```python
from build123d import *

# Parameters (mm, degrees)
F1_DEPTH  = 280
F2_R      = 4.25
F3_DEPTH  = 5.001
F4_R      = 2
F5_R      = 4.25
F6_DEPTH  = 5.001
F7_R      = 5
F8_W      = 10
F8_H      = 90
F9_DEPTH  = 40
F11_DEPTH = 145.001
F13_DEPTH = 5.001
F14_R     = 2


with BuildPart() as f1:
    # F0 (on Right) → F1 (new body)
    with BuildSketch(Plane.YZ):
        Polygon((0, -90), (0, 90), (-5, 90), (-5, -85), (-80, -85), (-80, -90), align=None)
    extrude(amount=F1_DEPTH)

    # F2 (on face) → F3 (cut, through all)
    with BuildSketch(Plane.XZ.offset(5)):
        with Locations((25, 59)):
            Circle(F2_R)
        with Locations((25, -59)):
            Circle(F2_R)
        with Locations((250, -59)):
            Circle(F2_R)
        with Locations((250, 59)):
            Circle(F2_R)
    extrude(amount=-F3_DEPTH, mode=Mode.SUBTRACT)

    # F4
    f4_edges = [f1.edges().sort_by_distance(p)[0] for p in [
        (0, -2.5, 90),
        (280, -2.5, 90),
        (280, -80, -87.5),
        (0, -80, -87.5),
    ]]
    fillet(f4_edges, radius=F4_R)

    # F5 (on face) → F6 (cut, through all)
    with BuildSketch(Plane.XY.offset(-85)):
        with Locations((140, -60)):
            Circle(F5_R)
    extrude(amount=-F6_DEPTH, mode=Mode.SUBTRACT)

    # F7
    f7_edges = [f1.edges().sort_by_distance(p)[0] for p in [
        (140, 0, -90),
    ]]
    fillet(f7_edges, radius=F7_R)

    # F8 (on face) → F9 (join)
    with BuildSketch(Plane.XZ.offset(5)):
        with Locations((140, -40)):
            Rectangle(F8_W, F8_H)
    extrude(amount=F9_DEPTH)

    # F10 (on face) → F11 (cut, through all)
    with BuildSketch(Plane.YZ.offset(145)):
        Polygon((-45, -85), (-5, 5), (-45, 5), align=None)
    extrude(amount=-F11_DEPTH, mode=Mode.SUBTRACT)

    # F12 (on face) → F13 (cut, through all)
    with BuildSketch(Plane.XY.offset(-85)):
        with BuildLine():
            Line((2, -80), (120, -80))
            Line((120, -80), (0, -5))
            Line((0, -5), (0, -78))
            ThreePointArc((0, -78), (0.5857864376, -79.4142135624), (2, -80))
        make_face()
        with BuildLine():
            Line((280, -78), (280, -5))
            Line((280, -5), (160, -80))
            Line((160, -80), (278, -80))
            ThreePointArc((278, -80), (279.4142135624, -79.4142135624), (280, -78))
        make_face()
    extrude(amount=-F13_DEPTH, mode=Mode.SUBTRACT)

    # F14
    f14_edges = [f1.edges().sort_by_distance(p)[0] for p in [
        (67.5, -5, -85),
        (212.5, -5, -85),
    ]]
    fillet(f14_edges, radius=F14_R)


solid = f1.part
```
Input: part model. Units: mm. Frame: model coordinates. A direction names the side the tool comes from. Give positions to 0.01 mm unless a question says otherwise; leave off trailing zeros. Order: outer loops, then holes, each group sorted by start corner. A loop starts at its lowest first (then second) coordinate and runs counter-clockwise, first axis right, second up.
1. Section B-B on x = 140. Return the cut outline in (y, z).
Derived:
outline: (-80, -90) - (-64.25, -90) - (-64.25, -85) - (-80, -85) - close; (-55.75, -90) - (-5, -90) arc R5 ccw to (0, -85) - (0, 90) - (-5, 90) - (-5, 5) - (-45, -85) - (-55.75, -85) - close
2. Material intervals for L1, parallel to Z at x = 125.5, y = -8; L2, parallel to Z at x = 250, y = -3.1; L3, parallel to Y at x = 98.5, z = -77, sorted ascending.
Derived:
L1: z = -90 to -85
L2: z = -89.62 to -63.25, -54.75 to 54.75, 63.25 to 90
L3: y = -5 to 0
3. Section C-C on y = -60. Return the cut outline in (x, z).
Derived:
outline: (88, -90) - (135.75, -90) - (135.75, -85) - (88, -85) - close; (144.25, -90) - (192, -90) - (192, -85) - (144.25, -85) - close
4. Mould query, pull axis Y, two halves, no side actions, for faces 4 (the cylindrical face through (136.63, -62.59, -87.46)), 5 (the flat face through (135, -20, -51)), 6 (the flat face through (140.07, -25.28, -40.63)). Classes: released by +Y, released by -Y, zero draft, split by the parting line, or undercut.
Derived:
face 4: undercut
face 5: zero draft
face 6: released by -Y
5. Reachability of faces 1 (the flat face through (138, -51, -85)), 2 (the cylindrical face through (246.63, -2.54, 56.41)), 3 (the flat face through (145, -20, -51)) from +Z, -Z, +X, -X, +Y, -Y: full face, straight path, thin tool, end or side. Return the list, or none.
Derived:
face 1: +Z, -Y
face 2: +Y, -Y
face 3: +Z, +X, -Y
6. Pin query (flat end, axial travel): pin 1 (1.5 mm diameter, centred on x = 99.5, y = -58.5, fed in from +Z); pin 2 (10 mm diameter, centred on y = -18.5, z = -47, fed in from -X); pin 3 (12 mm diameter, centred on x = 155.5, z = -5, fed in from -Y). Return the tip coordinate at first contact, or that it passes through.
Derived:
pin 1: stops at z = -85
pin 2: stops at x = 135
pin 3: stops at y = -5
7. Section D-D on x = 25. Return the cut outline in (y, z) (3 decimals), and give its area (3 significant figures).
Derived:
outline: (-20.625, -90) - (-5, -90) arc R5 ccw to (0, -85) - (0, -63.25) - (-5, -63.25) - (-5, -83) arc R2 cw to (-7, -85) - (-20.625, -85) - close; (-5, -54.75) - (0, -54.75) - (0, 54.75) - (-5, 54.75) - close; (-5, 63.25) - (0, 63.25) - (0, 90) - (-5, 90) - close
area: 889 mm2
8. Section A-A on z = 59. Return the cut outline in (x, y), and give its area (4 significant figures).
Derived:
outline: (0, -5) - (20.75, -5) - (20.75, 0) - (0, 0) - close; (29.25, -5) - (245.75, -5) - (245.75, 0) - (29.25, 0) - close; (254.25, -5) - (280, -5) - (280, 0) - (254.25, 0) - close
area: 1,315 mm2
